Could you check a few things on this drawing? It's one solid part, dimensions in mm from its lowest x, y, z. Coordinates: 2 decimals unless noted, no trailing zeros. Order: outer loops, then holes, each group sorted by start corner. A loop starts at its lowest first (then second) coordinate and runs counter-clockwise, first axis right, second up. Notation, with made-up numbers: (46, 3.25) - (84, 3.25) arc R27 cw to (84, 38.25) - close; hole circle Ø6 at (66, -39.5). An arc over 180 degrees is marked (long way). Return JSON: item names as keys, results as strings. Group by question number.
1) Imagine slicing it at C-C (x = 0.65). Write out the boundary of the cut face in (y, z), and give its area (3 significant figures).
2) Imagine slicing it at D-D (z = 14.25). Write out the boundary of the cut face in (x, y).
3) Imagine slicing it at A-A (y = 28.5). Write out the boundary of the cut face in (x, z).
4) If we mould it in two halves opening along Y, with no side actions, what happens to the marked faces 1, 2 and 3? For each: pulls with the +Y half, pulls with the -Y half, needs draft (parallel to the pull), parting line crosses it, or undercut.
5) If I drill on line 1 along Y through (x, z) = (1.9, 10); line 2 along Y through (x, z) = (0.65, 14.75); line 3 along Z through (x, y) = (1.3, 6), over which ranges is the centre line in solid material (lowest first)?
6) For pin 1 Ø1 at (x, z) = (2, 17) entering from -Y, with a flat end and sliding along its axis, tell me the tip position at first contact or that it passes through.
7) Imagine slicing it at B-B (z = 10). Write out the boundary of the cut face in (x, y).
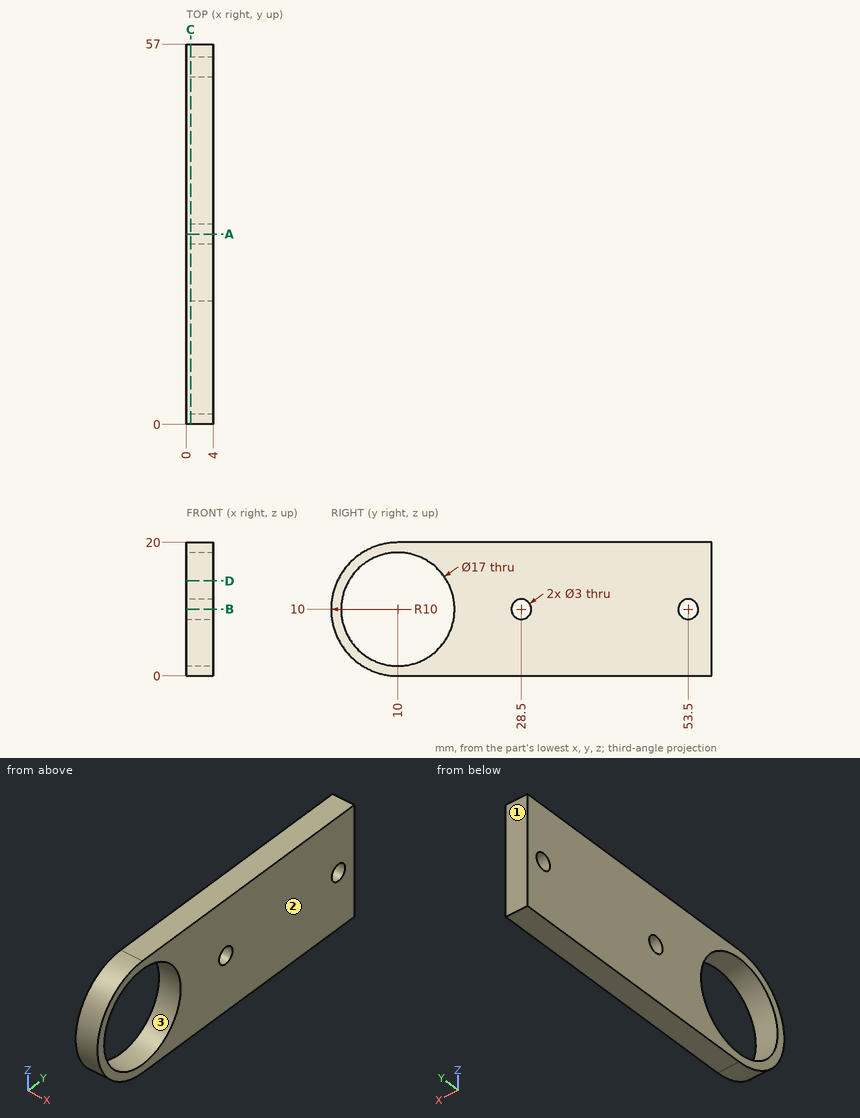
Calculated:
{
 "1": {"outline": "(10, 0) - (57, 0) - (57, 20) - (10, 20) arc R10 ccw to start; hole circle Ø17 at (10, 10); hole circle Ø3 at (28.5, 10); hole circle Ø3 at (53.5, 10)", "area": "856 mm2"},
 "2": {"outline": "(0, 0.95) - (4, 0.95) - (4, 2.64) - (0, 2.64) - close; (0, 17.36) - (4, 17.36) - (4, 57) - (0, 57) - close"},
 "3": {"outline": "(0, 0) - (4, 0) - (4, 8.5) - (0, 8.5) - close; (0, 11.5) - (4, 11.5) - (4, 20) - (0, 20) - close"},
 "4": {"face 1": "pulls with the +Y half", "face 2": "needs draft", "face 3": "undercut"},
 "5": {"line 1": "0 to 1.5, 18.5 to 27, 30 to 52, 55 to 57", "line 2": "1.2 to 2.95, 17.05 to 57", "line 3": "0.83 to 2.5, 17.5 to 19.17"},
 "6": {"pin 1": "y = 2.4"},
 "7": {"outline": "(0, 0) - (4, 0) - (4, 1.5) - (0, 1.5) - close; (0, 18.5) - (4, 18.5) - (4, 27) - (0, 27) - close; (0, 30) - (4, 30) - (4, 52) - (0, 52) - close; (0, 55) - (4, 55) - (4, 57) - (0, 57) - close"}
}
